Geometry check sheet. Reference: drawing and pictorial views, mm from the part's lowest x, y, z. A direction names the side the tool comes from. Coordinates: 2 decimals unless noted, no trailing zeros. Write each loop counter-clockwise with the first axis right and the second up, starting at its lowest first coordinate (ties: lowest second). Pieces come first, ordered by that corner, then holes. Notation, with made-up numbers: M -28,75 L 15,75 A20 cw 15,108 Z; hole C 74,44.25 d11. An arc over 180 degrees is marked long. One line per item, written item: value.
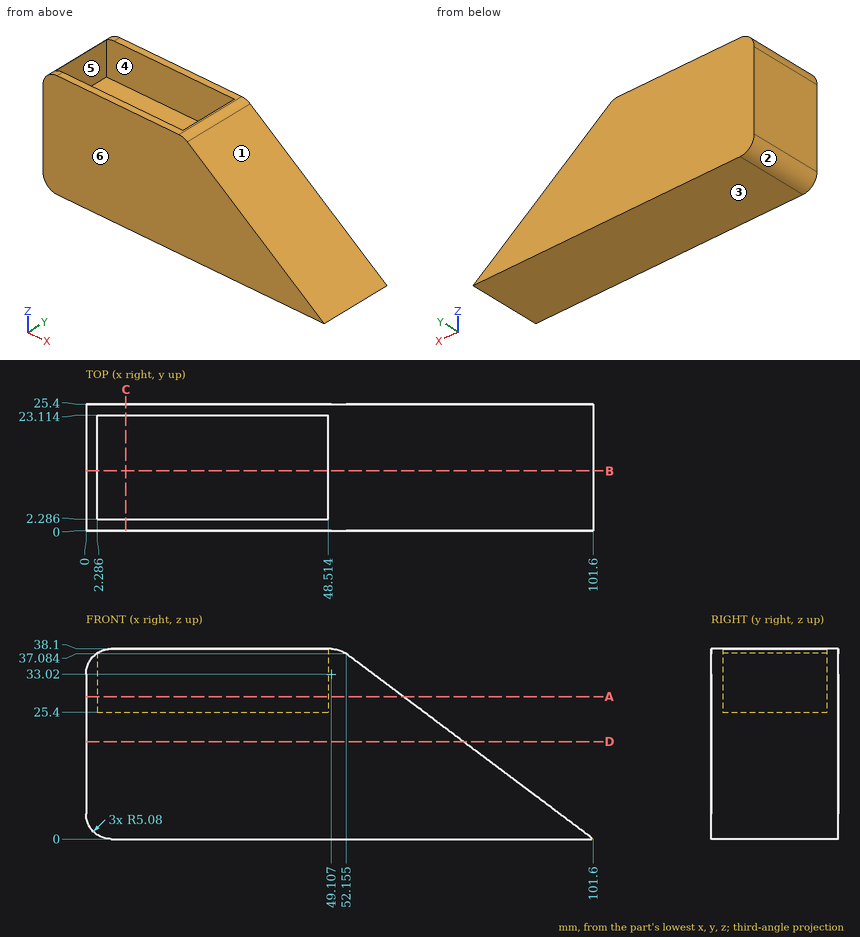
Item 1: Cross-section at B-B, the plane y = 12. Enter the section's corners in (x, z) (1 decimal), and give its area (3 significant figures).
The answers:
outline: M 0,5.1 A5.1 ccw 5.1,0 L 101.6,0 L 52.2,37.1 A5.1 ccw 49.1,38.1 L 48.5,38.1 L 48.5,25.4 L 2.3,25.4 L 2.3,37.3 A5.1 ccw 0,33 Z
area: 2,310 mm²
Item 2: Draft check along X on the marked faces 1, 2, 3 and 4. Enter one of: released by +X, released by -X, zero draft, split by the parting line, or undercut.
The answers:
face 1: released by +X
face 2: released by -X
face 3: zero draft
face 4: undercut
Item 3: Access from +Z, -Z, +X, -X, +Y, -Y to the whole of each face (thin tool, end or side, straight path). Record for the marked faces 5 and 6.
The answers:
face 5: +Z
face 6: +Z, -Z, +X, -X, -Y
Item 4: Go/stop test with flat-tipped pins: P1, Ø8, axis at y = 4.5, z = 27, coming from the +X side (1 decimal); P2, Ø3.5, axis at y = 17.5, z = 33, coming from the +X side (1 decimal); P3, Ø4, axis at y = 9, z = 12.5, coming from the +X side. Record where each tip stops, or that it passes through.
The answers:
P1: stops at x = 70.9
P2: stops at x = 59.9
P3: stops at x = 87.6
Item 5: Cross-section at C-C, the plane x = 8. Enter the section's corners in (y, z), and give its area (3 significant figures).
The answers:
outline: M 0,0 L 25.4,0 L 25.4,38.1 L 23.11,38.1 L 23.11,25.4 L 2.29,25.4 L 2.29,38.1 L 0,38.1 Z
area: 703 mm²
Item 6: Cross-section at D-D, the plane z = 19.5. Enter the section's corners in (x, y), and give its area (3 significant figures).
The answers:
outline: M 0,0 L 75.6,0 L 75.6,25.4 L 0,25.4 Z
area: 1,920 mm²
Item 7: Cross-section at A-A, the plane z = 28.5. Enter the section's corners in (x, y).
The answers:
outline: M 0,0 L 63.6,0 L 63.6,25.4 L 0,25.4 Z; hole M 2.29,2.29 L 48.51,2.29 L 48.51,23.11 L 2.29,23.11 Z
Item 8: Scan lines: line 1 (Y direction, x = 26, z = 32); line 2 (X direction, y = 21, z = 30.5) (1 decimal); line 3 (X direction, y = 4, z = 36.5) (1 decimal). Record each from-to range of solid material in increasing order.
The answers:
line 1: y = 0 to 2.29, 23.11 to 25.4
line 2: x = 0 to 2.3, 48.5 to 60.9
line 3: x = 1.4 to 2.3, 48.5 to 52.9
